Autodesk Inventor part; units mm, degrees
ref_plane "YZ Plane" through (0, 0, 0) normal (1, 0, 0) x (0, 1, 0)
ref_plane "XZ Plane" through (0, 0, 0) normal (0, 1, 0) x (-1, 0, 0)
ref_plane "XY Plane" through (0, 0, 0) normal (0, 0, 1) x (1, 0, 0)
ref_plane "Work Plane7" through (-1576.3187, -383.5702, 1516.5612) normal (0, 0, 1) x (1, 0, 0)
sketch "Sketch7" plane through (-1576.3187, -383.5702, 1516.5612) normal (0, 0, 1) x (1, 0, 0)
  arc A0 (159.3276, -330.8443) -> (156.2977, -331.6006) centre (159.7307, -338.9062) ccw
  arc A1 (156.2977, -331.6006) -> (153.9729, -333.2489) centre (159.7307, -338.9062) ccw
  arc A2 (153.9729, -333.2489) -> (153.7336, -335.2986) centre (162.867, -335.3261) ccw
  arc A3 (153.7336, -335.2986) -> (153.966, -337.3737) centre (162.867, -335.3261) ccw
  arc A4 (153.966, -337.3737) -> (154.5105, -337.975) centre (154.7761, -337.1873) ccw
  arc A5 (228.4965, -333.0839) -> (226.18, -331.4628) centre (222.6932, -338.9111) ccw
  arc A6 (228.4399, -337.3902) -> (228.4965, -333.0839) centre (220.1875, -335.1281) ccw
  arc A7 (227.7937, -337.975) -> (228.4399, -337.3902) centre (227.6994, -337.2214) ccw
  arc A8 (223.6782, -330.7382) -> (159.3276, -330.8443) centre (191.9649, -610.889) ccw
  arc A9 (226.18, -331.4628) -> (223.6782, -330.7382) centre (222.5826, -339.2015) ccw
  arc A10 (150.5551, -338.1583) -> (153.392, -341.2915) centre (154.7761, -337.1873) ccw
  arc A11 (150.2336, -335.2881) -> (150.5551, -338.1583) centre (162.867, -335.3261) ccw
  arc A12 (150.8193, -331.5239) -> (150.2336, -335.2881) centre (162.867, -335.3261) ccw
  arc A13 (154.8092, -328.4329) -> (150.8193, -331.5239) centre (159.7307, -338.9062) ccw
  arc A14 (159.0274, -327.3556) -> (154.8092, -328.4329) centre (159.7307, -338.9062) ccw
  arc A15 (224.0974, -327.2633) -> (159.0274, -327.3556) centre (191.9649, -610.889) ccw
  arc A16 (227.6596, -328.2909) -> (224.0974, -327.2633) centre (222.5826, -339.2015) ccw
  arc A17 (231.6266, -331.3184) -> (227.6596, -328.2909) centre (222.6932, -338.9111) ccw
  arc A18 (231.8286, -338.2666) -> (231.6266, -331.3184) centre (220.1875, -335.1281) ccw
  arc A19 (228.2282, -341.4479) -> (231.8286, -338.2666) centre (227.6994, -337.2214) ccw
  line L0 (153.392, -341.2915) -> (154.5105, -337.975)
  line L1 (227.7937, -337.975) -> (228.2282, -341.4479)
  point P0 (1576.3187, 383.5702)
  dimension "d20" = 73.2832
  dimension "d21" = 3.5
  dimension "d22" = 74.8362
extrude "Extrusion3" add sketch "Sketch7" along normal blind 20
properties part number "_3DPrint"
Part model, mm, in its own coordinate system. A direction names the side the tool comes from. Give positions to 0.01 mm unless a question says otherwise; leave off trailing zeros. Loops run counter-clockwise (first coordinate to the right, second up) from the corner with the lowest first, then second, coordinate; pieces in that order, holes last. Notation, with made-up numbers: M 53,-13.75 L 70,-13.75 A30 ccw 70,15.25 Z; hole C 12.25,88 d7. An arc over 180 degrees is marked long. Return JSON: item names as keys, results as strings.
1) Drill centre lines: line 1 (X direction, y = -718.75, z = 1533.5); line 2 (X direction, y = -722.75, z = 1532); line 3 (Y direction, x = -1367, z = 1532). Where is each one in solid material? Low to high.
Calculated:
{"line 1": "x = -1426.08 to -1422.58, -1347.57 to -1344.07", "line 2": "x = -1425.39 to -1422.21, -1348.37 to -1344.84", "line 3": "y = -713.05 to -709.55"}
2) Saw through at A-A, the plane z = 1520. List the corners of the cut face in (x, y) (1 decimal).
Calculated:
{"outline": "M -1426.1,-718.9 A12.6 ccw -1425.8,-721.7 A4.3 ccw -1422.9,-724.9 L -1421.8,-721.5 A0.8 cw -1422.4,-720.9 A9.1 cw -1422.6,-718.9 A9.1 cw -1422.3,-716.8 A8.1 cw -1420,-715.2 A8.1 cw -1417,-714.4 A281.9 cw -1352.6,-714.3 A8.5 cw -1350.1,-715 A8.2 cw -1347.8,-716.7 A8.6 cw -1347.9,-721 A0.8 cw -1348.5,-721.5 L -1348.1,-725 A4.3 ccw -1344.5,-721.8 A12.1 ccw -1344.7,-714.9 A11.7 ccw -1348.7,-711.9 A12 ccw -1352.2,-710.8 A285.4 ccw -1417.3,-710.9 A11.6 ccw -1421.5,-712 A11.6 ccw -1425.5,-715.1 A12.6 ccw Z"}
3) Saw through at D-D, the plane y = -719.75. List the corners of the cut face in (x, z), then the cut area to 3 significant figures.
Calculated:
{"outline": "M -1426.06,1516.56 L -1422.55,1516.56 L -1422.55,1536.56 L -1426.06,1536.56 Z; M -1347.64,1516.56 L -1344.12,1516.56 L -1344.12,1536.56 L -1347.64,1536.56 Z", "area": "141 mm2"}
4) Flat gauge pins, fed straight in: pin 1 Ø1 at (y, z) = (-722, 1527.5) entering from +X; pin 2 Ø5 at (x, z) = (-1370, 1532) entering from +Y; pin 3 Ø8 at (x, z) = (-1411, 1519.5) entering from +Y. Where does each tip first touch, or does it go through?
Calculated:
{"pin 1": "stops at x = -1344.4", "pin 2": "stops at y = -709.27", "pin 3": "stops at y = -709.92"}
5) Saw through at C-C, the plane x = -1399.5. List the corners of the cut face in (y, z).
Calculated:
{"outline": "M -712.93,1516.56 L -709.42,1516.56 L -709.42,1536.56 L -712.93,1536.56 Z"}
6) 3-axis set-ups, long thin cutter, end or side, ignore diameter. For faces 4 (the face through (-1348.93, -715.73, 1526.42)), 5 (the face through (-1385, -712, 1536.561)), 6 (the face through (-1351.38, -714.57, 1526.42)): which of +Z, -Z, +X, -X, +Y, -Y reach the whole face in a straight line?
Calculated:
{"face 4": "+Z, -Z", "face 5": "+Z, +X, -X, +Y, -Y", "face 6": "+Z, -Z, -Y"}
7) Pull direction X, two halves, no side cores. Call faces 1 (the face through (-1426.004, -720.323, 1526.421)), 2 (the face through (-1346.54, -713.14, 1526.42)), 3 (the face through (-1421.27, -715.9, 1526.42)): released by +X, released by -X, zero draft, split by the parting line, or undercut.
Calculated:
{"face 1": "released by -X", "face 2": "released by +X", "face 3": "undercut"}
8) Saw through at B-B, the plane y = -723.25. List the corners of the cut face in (x, z), then the cut area to 3 significant figures.
Calculated:
{"outline": "M -1425.08,1516.56 L -1422.38,1516.56 L -1422.38,1536.56 L -1425.08,1536.56 Z; M -1348.31,1516.56 L -1345.14,1516.56 L -1345.14,1536.56 L -1348.31,1536.56 Z", "area": "117 mm2"}
